from build123d import *

# Parameters (mm, degrees)
F0_R     = 11
F1_DEPTH = 5


with BuildPart() as f1:
    # F0 (on Top) → F1 (new body)
    with BuildSketch(Plane.XY):
        with BuildLine():
            ThreePointArc((33.682458, -2.5), (14, 0), (33.682458, 2.5))
            ThreePointArc((33.682458, 2.5), (34.394205, 1.418861), (35.61895, 1))
            Line((35.61895, 1), (36.649111, 1))
            ThreePointArc((36.649111, 1), (38.21804, 1.759653), (38.595128, 3.461538))
            ThreePointArc((38.595128, 3.461538), (30.240785, 13.64011), (17.076923, 13.306803))
            ThreePointArc((17.076923, 13.306803), (7.430987, 13.535462), (2.468312, 21.810015))
            ThreePointArc((2.468312, 21.810015), (-4.273896, 32.573046), (-16.855466, 34.306331))
            ThreePointArc((-16.855466, 34.306331), (-18.126104, 33.125515), (-17.996029, 31.395797))
            Line((-17.996029, 31.395797), (-17.480949, 30.503651))
            ThreePointArc((-17.480949, 30.503651), (-16.505832, 29.652422), (-15.213665, 29.5766))
            ThreePointArc((-15.213665, 29.5766), (-7.537499, 11.281092), (-19.543792, 27.0766))
            ThreePointArc((-19.543792, 27.0766), (-18.963372, 28.233561), (-19.213, 29.503651))
            Line((-19.213, 29.503651), (-19.72808, 30.395797))
            ThreePointArc((-19.72808, 30.395797), (-21.170423, 31.374703), (-22.832843, 30.850328))
            ThreePointArc((-22.832843, 30.850328), (-27.470574, 18.525969), (-20.59999, 7.292384))
            ThreePointArc((-20.59999, 7.292384), (-15.870723, -0.606189), (-19.600953, -9.022768))
            ThreePointArc((-19.600953, -9.022768), (-26.471536, -20.256353), (-21.833806, -32.580712))
            ThreePointArc((-21.833806, -32.580712), (-20.171385, -33.105087), (-18.729042, -32.126181))
            Line((-18.729042, -32.126181), (-18.213962, -31.234036))
            ThreePointArc((-18.213962, -31.234036), (-17.964334, -29.963945), (-18.544754, -28.806985))
            ThreePointArc((-18.544754, -28.806985), (-6.538462, -13.011476), (-14.214627, -31.306985))
            ThreePointArc((-14.214627, -31.306985), (-15.506794, -31.382806), (-16.481911, -32.234036))
            Line((-16.481911, -32.234036), (-16.996991, -33.126181))
            ThreePointArc((-16.996991, -33.126181), (-17.123577, -34.86474), (-15.838245, -36.04225))
            ThreePointArc((-15.838245, -36.04225), (-2.846172, -33.896463), (3.447106, -22.329571))
            ThreePointArc((3.447106, -22.329571), (7.922837, -14.284619), (17.076923, -13.306803))
            ThreePointArc((17.076923, -13.306803), (30.240785, -13.64011), (38.595128, -3.461538))
            ThreePointArc((38.595128, -3.461538), (38.21804, -1.759653), (36.649111, -1))
            Line((36.649111, -1), (35.61895, -1))
            ThreePointArc((35.61895, -1), (34.394205, -1.418861), (33.682458, -2.5))
        make_face()
        Circle(F0_R, mode=Mode.SUBTRACT)
    extrude(amount=F1_DEPTH)


solid = f1.part
For this review, take the finished solid that the model builds, in its own axes (mm). A direction names the side the tool comes from. Round coordinates to 2 decimals unless told otherwise and drop trailing zeros. Order: outer loops, then holes, each group sorted by start corner. A loop starts at its lowest first (then second) coordinate and runs counter-clockwise, first axis right, second up. Notation, with made-up numbers: (20.5, -28.75) -> (29.5, -28.75) arc R10 cw to (29.5, -12.75) -> close; hole circle Ø11 at (-17, 28). An arc over 180 degrees is marked (long way). Write item = value, one per line. Start each with the question number.
1) Tool access review of faces 4 (the face through (38.234, -1.78, 2.465)), 5 (the face through (34.409, -1.408, 2.465)): name each direction out of +Z, -Z, +X, -X, +Y, -Y from which nothing blocks a thin tool from reaching the whole face with its end or side.
2) Take a section at C-C on y = -6.5. State the section outline as (x, z) points, plus the area to 3 significant figures.
3) Take a section at A-A on x = 24. State the section outline as (y, z) points.
4) Insertion check: pin 1 (23 mm diameter, centred on x = -12.54, y = 19.94, fed in from +Z); pin 2 (0.8 mm diameter, centred on x = 36, z = 3, fed in from +Y); pin 3 (1.1 mm diameter, centred on x = 36.5, z = 1.5, fed in from -Y). Each pin has a flat end and moves straight along its axis. Give the tip position at first contact, or say it passes through.
5) Take a section at B-B on y = -30. State the section outline as (x, z) points, plus the area to 3 significant figures.
6) The part is to be moulded in two halves that separate along Y. For faces 1 (the face through (30.41, 13.56, 2.46)), 2 (the face through (0.5, -11.3, 0)), 3 (the face through (-15.49, -31.376, 2.465)), say which applies: +Y half, -Y half, draft (parallel to the pull), parting line (faces both ways), or undercut.
7) To check wall thickness, follow line 1 (X direction, y = 3.5, z = 3); line 2 (Y direction, x = 24, z = 3.9); line 3 (Y direction, x = -3.5, z = 1.2). State the ranges of each line that lie inside material, in increasing order. Write a range as from..to.
Verdict:
q1.face_4 = +Z, -Z, +X
q1.face_5 = +Z, -Z
q2.outline = (-17.36, 0) -> (-8.87, 0) -> (-8.87, 5) -> (-17.36, 5) -> close; (8.87, 0) -> (16.4, 0) -> (16.4, 5) -> (8.87, 5) -> close; (31.6, 0) -> (37.52, 0) -> (37.52, 5) -> (31.6, 5) -> close
q2.area = 110 mm2
q3.outline = (-15, 0) -> (-10, 0) -> (-10, 5) -> (-15, 5) -> close; (10, 0) -> (15, 0) -> (15, 5) -> (10, 5) -> close
q4.pin_1 = 5
q4.pin_2 = 9.51
q4.pin_3 = -9.07
q5.outline = (-24.01, 0) -> (-17.96, 0) -> (-17.96, 5) -> (-24.01, 5) -> close; (-6, 0) -> (0.94, 0) -> (0.94, 5) -> (-6, 5) -> close
q5.area = 65.0 mm2
q6.face_1 = +Y half
q6.face_2 = draft
q6.face_3 = undercut
q7.line_1 = -17.03..-10.43, 10.43..14.63, 33.37..38.59
q7.line_2 = -15..-10, 10..15
q7.line_3 = -34.34..-27.62, -15.72..-10.43, 10.43..15.66, 24.22..32.04
